Verification items for the finished model (mm, model axes). Coordinates: 2 decimals unless noted, no trailing zeros. Loops run counter-clockwise (first coordinate to the right, second up) from the corner with the lowest first, then second, coordinate; pieces in that order, holes last. Notation, with made-up numbers: (20.25, -3.5) -> (67.25, -3.5) arc R19 cw to (67.25, 5.5) -> close; hole circle Ø8 at (-35.75, 57). An arc over 180 degrees is marked (long way). Write item = value, one per line.
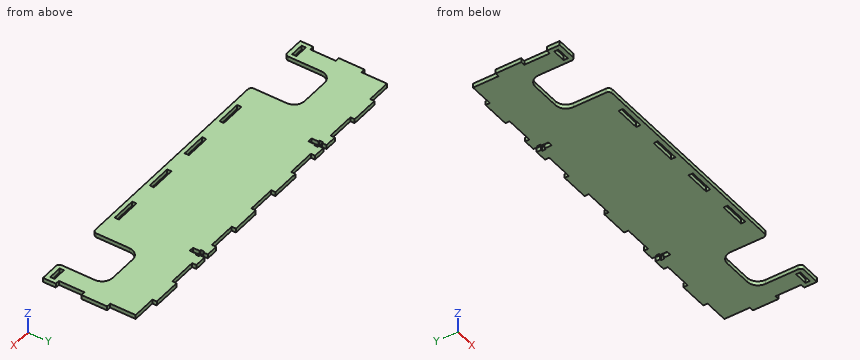
```python
from build123d import *

# Parameters (mm, degrees)
BOSS_EXTRUDE1_DEPTH     = 3
SKETCH2_W               = 3
SKETCH2_H               = 18
SKETCH2_W_2             = 17.666666666
SKETCH2_H_2             = 3
SKETCH2_W_3             = 17.666666667
SKETCH2_W_4             = 9.5
SKETCH2_W_5             = 20
CUT_EXTRUDE1_DEPTH      = 1
CUT_EXTRUDE1_DEPTH_BACK = 4
SKETCH3_W               = 3.2
SKETCH3_H               = 10.5
SKETCH3_W_2             = 5.2
SKETCH3_H_2             = 2.5
CUT_EXTRUDE2_DEPTH      = 1
CUT_EXTRUDE2_DEPTH_BACK = 4
FILLET1_R               = 7.5
FILLET2_R               = 2.5


with BuildPart() as part:
    # Sketch1 → Boss-Extrude1 (new body)
    with BuildSketch(Plane.XY):
        Polygon((-130, 33), (130, 33), (130, -33), (114.5, -33), (114.5, 0), (79.5, 0), (79.5, -33), (-79.5, -33), (-79.5, 0), (-114.5, 0), (-114.5, -33), (-130, -33), align=None)
    extrude(amount=BOSS_EXTRUDE1_DEPTH)

    # Sketch2 → Cut-Extrude1 (cut, two sides)
    with BuildSketch(Plane.XY.offset(3)) as cut_extrude1_sk:
        with Locations((-128.5, 21)):
            Rectangle(SKETCH2_W, SKETCH2_H)
        with Locations((-128.5, -15)):
            Rectangle(SKETCH2_W, SKETCH2_H)
        with Locations((-53, -28.5)):
            Rectangle(SKETCH2_W_2, SKETCH2_H_2)
        with Locations((-17.666666666, -28.5)):
            Rectangle(SKETCH2_W_3, SKETCH2_H_2)
        with Locations((17.666666666, -28.5)):
            Rectangle(SKETCH2_W_3, SKETCH2_H_2)
        with Locations((53, -28.5)):
            Rectangle(SKETCH2_W_2, SKETCH2_H_2)
        with Locations((122.25, -28.5)):
            Rectangle(SKETCH2_W_4, SKETCH2_H_2)
        with Locations((128.5, -15)):
            Rectangle(SKETCH2_W, SKETCH2_H)
        with Locations((128.5, 21)):
            Rectangle(SKETCH2_W, SKETCH2_H)
        Polygon((130, 33), (110, 33), (110, 30), (127, 30), (130, 30), align=None)
        with Locations((80, 31.5)):
            Rectangle(SKETCH2_W_5, SKETCH2_H_2)
        with Locations((40, 31.5)):
            Rectangle(SKETCH2_W_5, SKETCH2_H_2)
        with Locations((-40, 31.5)):
            Rectangle(SKETCH2_W_5, SKETCH2_H_2)
        with Locations((-80, 31.5)):
            Rectangle(SKETCH2_W_5, SKETCH2_H_2)
        with Locations((0, 31.5)):
            Rectangle(SKETCH2_W_5, SKETCH2_H_2)
        with Locations((-120, 31.5)):
            Rectangle(SKETCH2_W_5, SKETCH2_H_2)
        with Locations((-122.25, -28.5)):
            Rectangle(SKETCH2_W_4, SKETCH2_H_2)
    extrude(amount=CUT_EXTRUDE1_DEPTH, mode=Mode.SUBTRACT)
    extrude(cut_extrude1_sk.sketch, amount=-CUT_EXTRUDE1_DEPTH_BACK, mode=Mode.SUBTRACT)

    # Sketch3 → Cut-Extrude2 (cut, two sides)
    with BuildSketch(Plane.XY.offset(3)) as cut_extrude2_sk:
        with Locations((-60, 27.75)):
            Rectangle(SKETCH3_W, SKETCH3_H)
        with Locations((60, 27.75)):
            Rectangle(SKETCH3_W, SKETCH3_H)
        with Locations((-60, 28.575)):
            Rectangle(SKETCH3_W_2, SKETCH3_H_2)
        with Locations((60, 28.575)):
            Rectangle(SKETCH3_W_2, SKETCH3_H_2)
    extrude(amount=CUT_EXTRUDE2_DEPTH, mode=Mode.SUBTRACT)
    extrude(cut_extrude2_sk.sketch, amount=-CUT_EXTRUDE2_DEPTH_BACK, mode=Mode.SUBTRACT)

    # Fillet1
    fillet1_edges = [part.edges().sort_by_distance(p)[0] for p in [
        (114.5, 0, 1.5),
        (79.5, 0, 1.5),
        (-79.5, 0, 1.5),
        (-114.5, 0, 1.5),
    ]]
    fillet(fillet1_edges, radius=FILLET1_R)

    # Fillet2
    fillet2_edges = [part.edges().sort_by_distance(p)[0] for p in [
        (114.5, -33, 1.5),
        (79.5, -33, 1.5),
        (-79.5, -33, 1.5),
        (-114.5, -33, 1.5),
    ]]
    fillet(fillet2_edges, radius=FILLET2_R)


solid = part.part
```
1) Material ranges on line 1 (X direction, y = -19, z = 2.7); line 2 (Y direction, x = 15.5, z = 1.15); line 3 (Y direction, x = 7.5, z = 0.65), recorded low to high.
Ans:
line_1 = -127 to -114.5, -79.5 to 79.5, 114.5 to 127
line_2 = -33 to -30, -27 to 33
line_3 = -33 to 30
2) Depth check by flat-ended pin: pin 1 Ø1 at (y, z) = (-12.5, 2) entering from -X; pin 2 Ø0.9 at (x, z) = (-128, 1.5) entering from +Y; pin 3 Ø10 at (x, y) = (98, -9.5) entering from +Z; pin 4 Ø1.5 at (x, z) = (120.5, 1.5) entering from +Y. Enter the tip coordinate at first touch or a pass-through.
Ans:
pin_1 = -127
pin_2 = 12
pin_3 = through
pin_4 = 30
3) Sectioned sample at C-C, the plane y = 25. Record the cut outline in (x, z), plus the area to 3 significant figures.
Ans:
outline = (-127, 0) -> (-61.6, 0) -> (-61.6, 3) -> (-127, 3) -> close; (-58.4, 0) -> (58.4, 0) -> (58.4, 3) -> (-58.4, 3) -> close; (61.6, 0) -> (127, 0) -> (127, 3) -> (61.6, 3) -> close
area = 743 mm2
4) Sectioned sample at D-D, the plane z = 1.3. Count the separate pieces of the cut face and the enclosed holes in it, plus the area to 3 significant figures.
Ans:
separate_pieces = 1
enclosed_holes = 6
area = 13,900 mm2
5) Sectioned sample at B-B, the plane x = 53. Record the cut outline in (y, z).
Ans:
outline = (-33, 0) -> (-30, 0) -> (-30, 3) -> (-33, 3) -> close; (-27, 0) -> (33, 0) -> (33, 3) -> (-27, 3) -> close
6) Sectioned sample at A-A, the plane y = -15.5. Record the cut outline in (x, z), plus the area to 3 significant figures.
Ans:
outline = (-127, 0) -> (-114.5, 0) -> (-114.5, 3) -> (-127, 3) -> close; (-79.5, 0) -> (79.5, 0) -> (79.5, 3) -> (-79.5, 3) -> close; (114.5, 0) -> (127, 0) -> (127, 3) -> (114.5, 3) -> close
area = 552 mm2
